from build123d import *

# Parameters (mm, degrees)
SKETCH1_W           = 55
SKETCH1_H           = 8
BOSS_EXTRUDE1_DEPTH = 3
SKETCH2_R           = 1.5
SKETCH2_R_2         = 2.5
CUT_EXTRUDE1_DEPTH  = 4
SKETCH3_R           = 2
BOSS_EXTRUDE2_DEPTH = 10


with BuildPart() as part:
    # Sketch1 → Boss-Extrude1 (new body)
    with BuildSketch(Plane.XY):
        with Locations((27.5, 4)):
            Rectangle(SKETCH1_W, SKETCH1_H)
    extrude(amount=BOSS_EXTRUDE1_DEPTH)

    # Sketch2 → Cut-Extrude1 (cut, through all)
    with BuildSketch(Plane.XY.offset(3)):
        with Locations((13.97, 4)):
            Circle(SKETCH2_R)
        with Locations((20.5, 4)):
            Circle(SKETCH2_R)
        with Locations((41.03, 4)):
            Circle(SKETCH2_R)
        with Locations((34.5, 4)):
            Circle(SKETCH2_R)
        with Locations((27.5, 4)):
            Circle(SKETCH2_R_2)
    extrude(amount=-CUT_EXTRUDE1_DEPTH, mode=Mode.SUBTRACT)

    # Sketch3 → Boss-Extrude2 (add)
    with BuildSketch(Plane.XY):
        with Locations((51.725977791, 4)):
            Circle(SKETCH3_R)
        with Locations((3.013958935, 4)):
            Circle(SKETCH3_R)
    extrude(amount=BOSS_EXTRUDE2_DEPTH)


solid = part.part
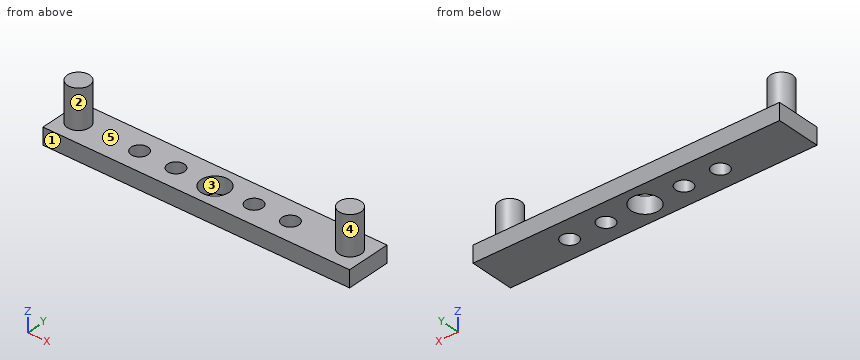
Design review of the part built by this model. Coordinates are the model's own, in mm. Face numbers are marked on the shaded views. A direction names the side the tool comes from. Coordinates: 2 decimals unless noted, no trailing zeros. Order: outer loops, then holes, each group sorted by start corner. A loop starts at its lowest first (then second) coordinate and runs counter-clockwise, first axis right, second up. Notation, with made-up numbers: (67.25, -27) -> (104.25, -27) arc R23 ccw to (104.25, -5) -> close; hole circle Ø2 at (-23, 42.5). An arc over 180 degrees is marked (long way). Use one line per item in the form item = value. Start each with the question number.
(1) Add section C-C on z = 1.75. State the section outline as (x, y) points.
(2) Add section D-D on x = 27.5. State the section outline as (y, z) points.
(3) Add section A-A on x = 13.97. State the section outline as (y, z) points, plus the area to 3 significant figures.
(4) For the marked faces 1 and 2, list the 3-axis set-ups (+Z, -Z, +X, -X, +Y, -Y) from which the entire face can be reached by the end or side of a thin tool; tool diameter is ignored.
(5) For probe 1 along Y at (x, z) = (34.5, 2.3); probe 2 along X at (y, z) = (3.5, 2.5); probe 3 along Y at (x, z) = (27.5, 1.75), list the stretches that pass through material, from the lowest coordinate up.
(6) Add section B-B on y = 4. Give the number of separate pieces and of enclosed holes in the cut face, plus the area to 3 significant figures.
(7) The part is to be moulded in two halves that separate along Y. For the marked faces 3, 4 and 5, say which applies: +Y half, -Y half, draft (parallel to the pull), parting line (faces both ways), or undercut.
(8) Insertion check: pin 1 (2.5 mm diameter, centred on x = 20.5, y = 4, fed in from +Z); pin 2 (4 mm diameter, centred on x = 29.5, y = 2, fed in from +Z). Each pin has a flat end and moves straight along its axis. Give the tip position at first contact, or say it passes through.
Answer block:
q1.outline = (0, 0) -> (55, 0) -> (55, 8) -> (0, 8) -> close; hole circle Ø3 at (13.97, 4); hole circle Ø3 at (20.5, 4); hole circle Ø5 at (27.5, 4); hole circle Ø3 at (34.5, 4); hole circle Ø3 at (41.03, 4)
q2.outline = (0, 0) -> (1.5, 0) -> (1.5, 3) -> (0, 3) -> close; (6.5, 0) -> (8, 0) -> (8, 3) -> (6.5, 3) -> close
q3.outline = (0, 0) -> (2.5, 0) -> (2.5, 3) -> (0, 3) -> close; (5.5, 0) -> (8, 0) -> (8, 3) -> (5.5, 3) -> close
q3.area = 15.0 mm²
q4.face_1 = +Z, -Z, +X, -X, -Y
q4.face_2 = +Z
q5.probe_1 = 0 to 2.5, 5.5 to 8
q5.probe_2 = 0 to 12.56, 15.38 to 19.09, 21.91 to 25.05, 29.95 to 33.09, 35.91 to 39.62, 42.44 to 55
q5.probe_3 = 0 to 1.5, 6.5 to 8
q6.separate_pieces = 6
q6.enclosed_holes = 0
q6.area = 170 mm²
q7.face_3 = undercut
q7.face_4 = parting line
q7.face_5 = draft
q8.pin_1 = through
q8.pin_2 = 3
